from build123d import *

# Parameters (mm, degrees)
F0_W      = 457.2
F0_H      = 203.2
F1_DEPTH  = 19.05
F2_W      = 203.2
F2_H      = 59.69
F3_R      = 10.414
F3_R_2    = 8.763
F3_R_3    = 8.382
F5_DEPTH  = 19.05
F6_W      = 87.63
F6_H      = 13.208
F11_DEPTH = 12.7
F8_W      = 161.29
F8_H      = 20.32
F8_W_2    = 203.2
F8_H_2    = 38.1
F8_H_3    = 40.64
F12_DEPTH = 12.7
F9_W      = 25.4
F9_H      = 152.4
F10_W     = 33.02
F10_H     = 63.5
F13_DEPTH = 12.7
F7_W      = 19.05
F7_H      = 157.48
F14_DEPTH = 12.7
F15_DEPTH = 12.7
F16_DEPTH = 12.7


# Not quite as in the source:
# - the program builds the solid bodies; features that only make, move or delete a surface that nothing else refers to are left out


with BuildPart() as f1:
    # F0 (on Top) → F1 (new body)
    with BuildSketch(Plane.XY):
        with Locations((-168.2645873785, 42.8677027285)):
            Rectangle(F0_W, F0_H)
    extrude(amount=F1_DEPTH)

    # F2 (on face) + F3 (on face) → F5 (join)
    with BuildSketch(Plane.XY.offset(19.05)):
        with Locations((-182.8039201736, 111.6589910698)):
            Rectangle(F2_W, F2_H)
    with BuildSketch(Plane.XY.offset(19.05)):
        with Locations((-337.6098275185, 94.2841172218)):
            Circle(F3_R)
        with Locations((-337.6098275185, 50.222992897)):
            Circle(F3_R_2)
        with Locations((-337.6098275185, 21.9573695213)):
            Circle(F3_R_3)
    extrude(amount=-F5_DEPTH)

    # F6 (on face) → F11 (cut)
    with BuildSketch(Plane.XY.offset(19.05)):
        with Locations((-340.3499591923, 122.5030114927)):
            Rectangle(F6_W, F6_H)
    extrude(amount=-F11_DEPTH, mode=Mode.SUBTRACT)

    # F8 (on face) → F12 (cut)
    with BuildSketch(Plane.XY.offset(19.05)):
        with Locations((-230.1238527489, 58.5634791589)):
            Rectangle(F8_W, F8_H)
        with Locations((-209.1688527489, 19.05)):
            Rectangle(F8_W_2, F8_H_2)
        with Locations((-209.1688527489, -23.6032848585)):
            Rectangle(F8_W_2, F8_H_3)
    extrude(amount=-F12_DEPTH, mode=Mode.SUBTRACT)

    # F9 (on face) + F10 (on face) → F13 (cut)
    with BuildSketch(Plane.XY.offset(19.05)):
        with Locations((-57.1830842316, 34.0140676022)):
            Rectangle(F9_W, F9_H)
    with BuildSketch(Plane.XY.offset(19.05)):
        with Locations((-8.2516423559, 9.3228359818)):
            Rectangle(F10_W, F10_H)
    extrude(amount=-F13_DEPTH, mode=Mode.SUBTRACT)

    # F7 (on face) → F14 (cut)
    with BuildSketch(Plane.XY.offset(19.05)):
        with Locations((26.3747599661, 61.2730749154)):
            Rectangle(F7_W, F7_H)
    extrude(amount=-F14_DEPTH, mode=Mode.SUBTRACT)

    # F2 (on face) → F15 (cut)
    with BuildSketch(Plane.XY.offset(19.05)):
        with Locations((-182.8039201736, 111.6589910698)):
            Rectangle(F2_W, F2_H)
    extrude(amount=-F15_DEPTH, mode=Mode.SUBTRACT)

    # F3 (on face) → F16 (cut)
    with BuildSketch(Plane.XY.offset(19.05)):
        with Locations((-337.6098275185, 94.2841172218)):
            Circle(F3_R)
        with Locations((-337.6098275185, 50.222992897)):
            Circle(F3_R_2)
        with Locations((-337.6098275185, 21.9573695213)):
            Circle(F3_R_3)
    extrude(amount=-F16_DEPTH, mode=Mode.SUBTRACT)


solid = f1.part
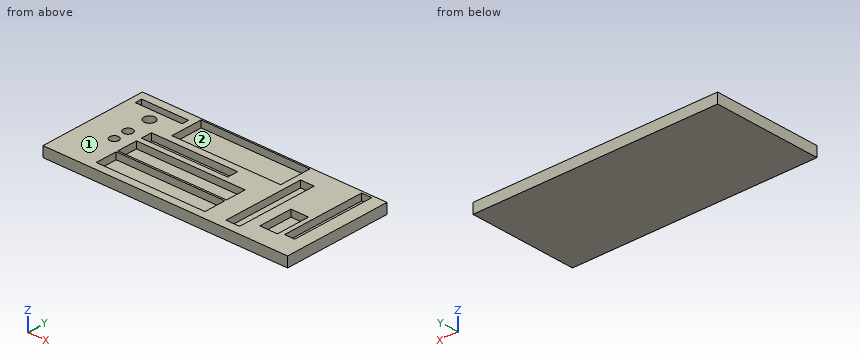
Design review of the part built by this model. Coordinates are the model's own, in mm. Face numbers are marked on the shaded views. Coordinates: 2 decimals unless noted, no trailing zeros. Order: outer loops, then holes, each group sorted by start corner. A loop starts at its lowest first (then second) coordinate and runs counter-clockwise, first axis right, second up. Notation, with made-up numbers: (68, -6.5) -> (119, -6.5) arc R21 ccw to (119, 3.5) -> close; hole circle Ø2 at (22, 88.25). An arc over 180 degrees is marked (long way). Use one line per item in the form item = value. Start each with the question number.
(1) The part is to be moulded in two halves that separate along X. For the marked faces 1 and 2, say which applies: +X half, -X half, draft (parallel to the pull), parting line (faces both ways), or undercut.
(2) For probe 1 along Y at (x, z) = (-208, 11.5); probe 2 along X at (y, z) = (8, 16.25); probe 3 along Y at (x, z) = (-89.5, 14.75), list the stretches that pass through material, from the lowest coordinate up.
(3) Insertion check: pin 1 (2 mm diameter, centred on x = -264.5, y = 53, fed in from +Z). The pin has a flat end and moves straight along its axis. Give the tip position at first contact, or say it passes through.
(4) Add section B-B on y = 74. State the section outline as (x, z) points.
(5) Add section D-D on z = 14.25. Give the number of separate pieces and of enclosed holes in the cut face, plus the area to 3 significant figures.
(6) Add section A-A on x = 1. State the section outline as (y, z) points.
(7) Add section C-C on x = -62. State the section outline as (y, z) points.
Answer block:
q1.face_1 = draft
q1.face_2 = undercut
q2.probe_1 = -58.73 to -43.92, -3.28 to 0, 38.1 to 48.4, 68.72 to 81.81, 141.5 to 144.47
q2.probe_2 = -396.86 to -310.77, -107.57 to -69.88, -44.48 to -24.76, 8.26 to 16.85, 35.9 to 60.34
q2.probe_3 = -58.73 to 81.81, 141.5 to 144.47
q3.pin_1 = 6.35
q4.outline = (-396.86, 0) -> (60.34, 0) -> (60.34, 19.05) -> (35.9, 19.05) -> (35.9, 6.35) -> (16.85, 6.35) -> (16.85, 19.05) -> (-44.48, 19.05) -> (-44.48, 6.35) -> (-69.88, 6.35) -> (-69.88, 19.05) -> (-396.86, 19.05) -> close
q5.separate_pieces = 1
q5.enclosed_holes = 11
q5.area = 50,600 mm²
q6.outline = (-58.73, 0) -> (144.47, 0) -> (144.47, 19.05) -> (41.07, 19.05) -> (41.07, 6.35) -> (-22.43, 6.35) -> (-22.43, 19.05) -> (-58.73, 19.05) -> close
q7.outline = (-58.73, 0) -> (144.47, 0) -> (144.47, 19.05) -> (110.21, 19.05) -> (110.21, 6.35) -> (-42.19, 6.35) -> (-42.19, 19.05) -> (-58.73, 19.05) -> close
